```python
from build123d import *

# Parameters (mm, degrees)
BOSS_EXTRUDE1_START         = -2.3876
BOSS_EXTRUDE1_DEPTH         = 4.7752
SKETCH4_R                   = 3.2639
CUT_EXTRUDE1_DEPTH          = 55.092721646
LPATTERN1_COUNT             = 3
LPATTERN1_PITCH             = 25.4
CIRPATTERN1_COPY_1_SKETCH_R = 3.2639
CIRPATTERN1_COPY_1_DEPTH    = 55.092721646
CIRPATTERN1_COPY_2_SKETCH_R = 3.2639
CIRPATTERN1_COPY_2_DEPTH    = 55.092721646
CIRPATTERN1_COPY_7_SKETCH_R = 3.2639
CIRPATTERN1_COPY_7_DEPTH    = 55.092721646
FILLET1_R                   = 1.27
FILLET2_R                   = 0.254


with BuildPart() as part:
    # Sketch3 → Boss-Extrude1 (new body)
    with BuildSketch(Plane.XY.offset(BOSS_EXTRUDE1_START)):
        Polygon((-38.1, 38.1), (-38.1, -38.1), (38.1, -38.1), (38.1, -12.7), (-12.7, 38.1), align=None)
    extrude(amount=BOSS_EXTRUDE1_DEPTH)

    # Sketch4 → Cut-Extrude1 (cut, symmetric)
    with BuildSketch(Plane.XY.offset(2.3876)):
        with Locations((-25.4, -25.4)):
            Circle(SKETCH4_R)
    cut_extrude1 = extrude(amount=CUT_EXTRUDE1_DEPTH, both=True, mode=Mode.SUBTRACT)

    # Cut-Extrude2 cone 1 section (through the dimple's axis) → Cut-Extrude2 (revolve, cut)
    with BuildSketch(Plane(origin=(-25.4, -25.4, 2.3876), x_dir=(0, -1, 0), z_dir=(1, 0, 0))):
        Polygon((0, 0), (3.7719, 0), (0, 3.7719), align=None)
    cut_extrude2 = revolve(axis=Axis((-25.4, -25.4, 2.3876), (0, 0, -1)), mode=Mode.SUBTRACT)

    # Cut-Extrude3 cone 1 section (through the dimple's axis) → Cut-Extrude3 (revolve, cut)
    with BuildSketch(Plane(origin=(-25.4, -25.4, -2.3876), x_dir=(0, 1, 0), z_dir=(1, 0, 0))):
        Polygon((0, 0), (3.7719, 0), (0, 3.7719), align=None)
    cut_extrude3 = revolve(axis=Axis((-25.4, -25.4, -2.3876), (0, 0, 1)), mode=Mode.SUBTRACT)

    # LPattern1: Cut-Extrude1, Cut-Extrude2, Cut-Extrude3 ×3
    with Locations(*[(0, i * LPATTERN1_PITCH, 0) for i in range(1, LPATTERN1_COUNT)]):
        add(cut_extrude1, mode=Mode.SUBTRACT)
        add(cut_extrude2, mode=Mode.SUBTRACT)
        add(cut_extrude3, mode=Mode.SUBTRACT)

    # CirPattern1 copy 1 sketch → CirPattern1 copy 1 (cut, symmetric)
    with BuildSketch(Plane(origin=(25.4, -50.8, 2.3876), x_dir=(0, -1, 0), z_dir=(0, 0, 1))):
        with Locations((-25.4, -25.4)):
            Circle(CIRPATTERN1_COPY_1_SKETCH_R)
    extrude(amount=CIRPATTERN1_COPY_1_DEPTH, both=True, mode=Mode.SUBTRACT)

    # CirPattern1 copy 2 sketch → CirPattern1 copy 2 (cut, symmetric)
    with BuildSketch(Plane(origin=(50.8, -50.8, 2.3876), x_dir=(0, -1, 0), z_dir=(0, 0, 1))):
        with Locations((-25.4, -25.4)):
            Circle(CIRPATTERN1_COPY_2_SKETCH_R)
    extrude(amount=CIRPATTERN1_COPY_2_DEPTH, both=True, mode=Mode.SUBTRACT)

    # CirPattern1 copy 3 sketch → CirPattern1 copy 3 (revolve, cut)
    with BuildSketch(Plane(origin=(0, -25.4, 2.3876), x_dir=(-1, 0, 0), z_dir=(0, -1, 0))):
        Polygon((0, 0), (3.7719, 0), (0, 3.7719), align=None)
    revolve(axis=Axis((0, -25.4, 2.3876), (0, 0, -1)), mode=Mode.SUBTRACT)

    # CirPattern1 copy 4 sketch → CirPattern1 copy 4 (revolve, cut)
    with BuildSketch(Plane(origin=(25.4, -25.4, 2.3876), x_dir=(-1, 0, 0), z_dir=(0, -1, 0))):
        Polygon((0, 0), (3.7719, 0), (0, 3.7719), align=None)
    revolve(axis=Axis((25.4, -25.4, 2.3876), (0, 0, -1)), mode=Mode.SUBTRACT)

    # CirPattern1 copy 5 sketch → CirPattern1 copy 5 (revolve, cut)
    with BuildSketch(Plane(origin=(0, -25.4, -2.3876), x_dir=(1, 0, 0), z_dir=(0, -1, 0))):
        Polygon((0, 0), (3.7719, 0), (0, 3.7719), align=None)
    revolve(axis=Axis((0, -25.4, -2.3876), (0, 0, 1)), mode=Mode.SUBTRACT)

    # CirPattern1 copy 6 sketch → CirPattern1 copy 6 (revolve, cut)
    with BuildSketch(Plane(origin=(25.4, -25.4, -2.3876), x_dir=(1, 0, 0), z_dir=(0, -1, 0))):
        Polygon((0, 0), (3.7719, 0), (0, 3.7719), align=None)
    revolve(axis=Axis((25.4, -25.4, -2.3876), (0, 0, 1)), mode=Mode.SUBTRACT)

    # CirPattern1 copy 7 sketch → CirPattern1 copy 7 (cut, symmetric)
    with BuildSketch(Plane(origin=(0, -50.8, 2.3876), x_dir=(0, -1, 0), z_dir=(0, 0, 1))):
        with Locations((-25.4, -25.4)):
            Circle(CIRPATTERN1_COPY_7_SKETCH_R)
    extrude(amount=CIRPATTERN1_COPY_7_DEPTH, both=True, mode=Mode.SUBTRACT)

    # CirPattern1 copy 8 sketch → CirPattern1 copy 8 (revolve, cut)
    with BuildSketch(Plane(origin=(-25.4, -25.4, 2.3876), x_dir=(-1, 0, 0), z_dir=(0, -1, 0))):
        Polygon((0, 0), (3.7719, 0), (0, 3.7719), align=None)
    revolve(axis=Axis((-25.4, -25.4, 2.3876), (0, 0, -1)), mode=Mode.SUBTRACT)

    # CirPattern1 copy 9 sketch → CirPattern1 copy 9 (revolve, cut)
    with BuildSketch(Plane(origin=(-25.4, -25.4, -2.3876), x_dir=(1, 0, 0), z_dir=(0, -1, 0))):
        Polygon((0, 0), (3.7719, 0), (0, 3.7719), align=None)
    revolve(axis=Axis((-25.4, -25.4, -2.3876), (0, 0, 1)), mode=Mode.SUBTRACT)

    # Fillet1
    fillet1_edges = [part.edges().sort_by_distance(p)[0] for p in [
        (-12.7, 38.1, 0),
        (38.1, -12.7, 0),
        (38.1, -38.1, 0),
        (-38.1, -38.1, 0),
        (-38.1, 38.1, 0),
    ]]
    fillet(fillet1_edges, radius=FILLET1_R)

    # Fillet2
    fillet2_edges = [part.edges().sort_by_distance(p)[0] for p in [
        (12.7, 12.7, -2.3876),
        (12.7, 12.7, 2.3876),
        (-25.028025612, 38.1, -2.3876),
        (38.1, -25.028025612, -2.3876),
        (0, -38.1, -2.3876),
        (-38.1, 0, -2.3876),
        (-12.740043265, 38.003327006, -2.3876),
        (-37.728025612, 37.728025612, -2.3876),
        (-37.728025612, -37.728025612, -2.3876),
        (37.728025612, -37.728025612, -2.3876),
        (38.003327006, -12.740043265, -2.3876),
        (38.1, -25.028025612, 2.3876),
        (-25.028025612, 38.1, 2.3876),
        (-38.1, 0, 2.3876),
        (0, -38.1, 2.3876),
        (-12.740043265, 38.003327006, 2.3876),
        (-37.728025612, 37.728025612, 2.3876),
        (-37.728025612, -37.728025612, 2.3876),
        (37.728025612, -37.728025612, 2.3876),
        (38.003327006, -12.740043265, 2.3876),
    ]]
    fillet(fillet2_edges, radius=FILLET2_R)


solid = part.part
```
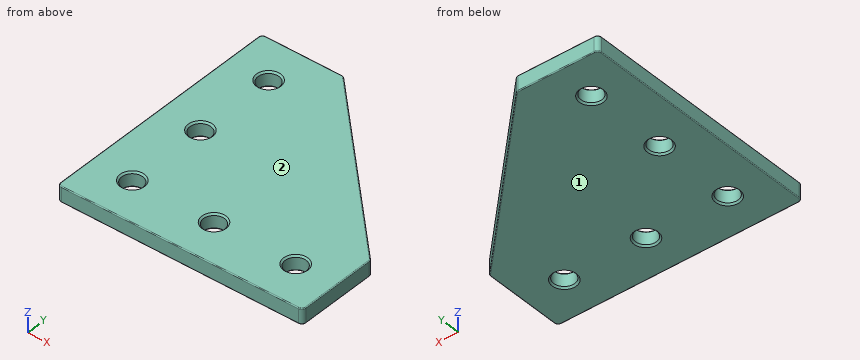
The listing builds one solid part. Answer for the finished solid, in the listing's coordinates (mm). Face numbers are marked on the shaded views. Coordinates: 2 decimals unless noted, no trailing zeros. Loops run counter-clockwise (first coordinate to the right, second up) from the corner with the lowest first, then second, coordinate; pieces in that order, holes last. Notation, with made-up numbers: (57.25, -21.5) - (116.25, -21.5) arc R32 cw to (116.25, 10.5) - close; hole circle Ø1 at (-22, -30). An arc over 180 degrees is marked (long way). Use a Markdown table: item, result. Add a question column.
1) Find the intervals of material crossed by line 1 (X direction, y = -25.4, z = -0.85); line 2 (Y direction, x = 0, z = -0.3), in increasing order.
2) The part is cut by section C-C, the plane z = -0.1. Give the vertices of the cut face in (x, y).
3) The mould has two halves that part along Z. Classify the marked faces 1 and 2: released by +Z, released by -Z, zero draft, split by the parting line, or undercut.
4) Given pin 1 (2 mm diameter, centred on x = 23, y = 2.5, fed in from +Z); pin 2 (6 mm diameter, centred on x = -25.4, y = 25.4, fed in from -Z); pin 3 (2 mm diameter, centred on y = -7, z = 1, fed in from +X); pin 4 (1.5 mm diameter, centred on y = 9, z = -0.5, fed in from +X), each flat-ended and moving along its own axis, determine where each tip first touches the part or whether it passes through.
5) The part is cut by section A-A, the plane y = -25.4. State how many separate pieces and enclosed holes the cut face has, and give its area (3 significant figures).
Here are the results:
| question | item | result |
|---|---|---|
| 1 | line 1 | x = -38.1 to -28.66, -22.14 to -3.26, 3.26 to 22.14, 28.66 to 38.1 |
| 1 | line 2 | y = -38.1 to -28.66, -22.14 to 25.4 |
| 2 | outline | (-38.1, -36.83) arc R1.27 ccw to (-36.83, -38.1) - (36.83, -38.1) arc R1.27 ccw to (38.1, -36.83) - (38.1, -13.23) arc R1.27 ccw to (37.73, -12.33) - (-12.33, 37.73) arc R1.27 ccw to (-13.23, 38.1) - (-36.83, 38.1) arc R1.27 ccw to (-38.1, 36.83) - close; hole circle Ø6.53 at (-25.4, -25.4); hole circle Ø6.53 at (-25.4, 0); hole circle Ø6.53 at (-25.4, 25.4); hole circle Ø6.53 at (0, -25.4); hole circle Ø6.53 at (25.4, -25.4) |
| 3 | face 1 | released by -Z |
| 3 | face 2 | released by +Z |
| 4 | pin 1 | stops at z = 2.39 |
| 4 | pin 2 | passes through |
| 4 | pin 3 | stops at x = 33.4 |
| 4 | pin 4 | stops at x = 17.15 |
| 5 | separate pieces | 4 |
| 5 | enclosed holes | 0 |
| 5 | area | 269 mm^2 |
